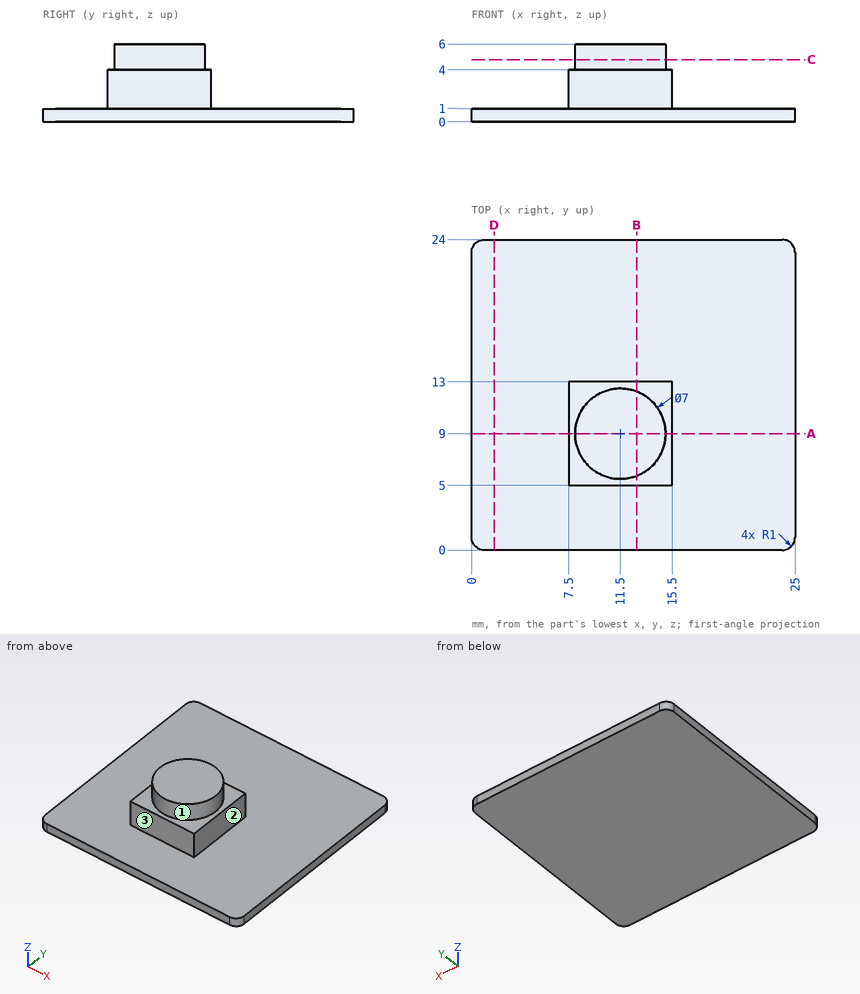
Can you work these out from the drawing? Everything is in mm from the part's minimum corner. A direction names the side the tool comes from. Coordinates: 2 decimals unless noted, no trailing zeros. Loops run counter-clockwise (first coordinate to the right, second up) from the corner with the lowest first, then second, coordinate; pieces in that order, holes last.
1) Imagine slicing it at D-D on x = 1.75. List the corners of the cut face in (y, z) for me.
2) Imagine slicing it at C-C on z = 4.8. List the corners of the cut face in (x, y) for me, plus the area to 3 significant figures.
3) Imagine slicing it at A-A on y = 9. List the corners of the cut face in (x, z) for me.
4) For pin 1 (0.9 mm diameter, centred on x = 13, z = 2.5, fed in from -Y); pin 2 (3 mm diameter, centred on x = 3, y = 9, fed in from +Z); pin 3 (3 mm diameter, centred on y = 2.5, z = 3.5, fed in from +X); pin 4 (0.9 mm diameter, centred on x = 13, z = 2.5, fed in from +Y), each with a flat end and sliding along its axis, tell me the tip position at first contact or that it passes through.
5) I need wall thicknesses on probe 1 along Y at (x, z) = (11.5, 2); probe 2 along X at (y, z) = (7.75, 3.75); probe 3 along Z at (x, y) = (18, 8.5). Which ranges of each line are inside material? Lowest first, please.
6) Imagine slicing it at B-B on x = 12.75. List the corners of the cut face in (y, z) for me, plus the area to 3 significant figures.
7) Which directions (+Z, -Z, +X, -X, +Y, -Y) give clear straight access to the entire face, cutting with the end or side of a thin tool? Please do the marked faces 1, 2 and 3.
Completed:
1. outline: (0, 0) - (24, 0) - (24, 1) - (0, 1) - close
2. outline: circle Ø7 at (11.5, 9)
2. area: 38.5 mm2
3. outline: (0, 0) - (25, 0) - (25, 1) - (15.5, 1) - (15.5, 4) - (15, 4) - (15, 6) - (8, 6) - (8, 4) - (7.5, 4) - (7.5, 1) - (0, 1) - close
4. pin 1: stops at y = 5
4. pin 2: stops at z = 1
4. pin 3: passes through
4. pin 4: stops at y = 13
5. probe 1: y = 5 to 13
5. probe 2: x = 7.5 to 15.5
5. probe 3: z = 0 to 1
6. outline: (0, 0) - (24, 0) - (24, 1) - (13, 1) - (13, 4) - (12.27, 4) - (12.27, 6) - (5.73, 6) - (5.73, 4) - (5, 4) - (5, 1) - (0, 1) - close
6. area: 61.1 mm2
7. face 1: +Z
7. face 2: +Z, +X, +Y, -Y
7. face 3: +Z, +X, -X, -Y
